```python
from build123d import *

# Parameters (mm, degrees)
SKETCH_1_W = 52
SKETCH_1_H = 6.25
SKETCH_4_W = 52
SKETCH_4_H = 4.25


with BuildPart() as part:
    # ｽｹｯﾁ1 → 回転1 (revolve)
    with BuildSketch(Plane.XY, mode=Mode.PRIVATE) as revolve_1_sk:
        with Locations((26, 3.125)):
            Rectangle(SKETCH_1_W, SKETCH_1_H)
    revolve(revolve_1_sk.sketch.rotate(Axis((500, 0, 0), (-1, 0, 0)), 270), axis=Axis((500, 0, 0), (-1, 0, 0)))

    # ｽｹｯﾁ2 → ｶｯﾄ - 回転1 (revolve, cut)
    with BuildSketch(Plane.XY, mode=Mode.PRIVATE) as cut_revolve_1_sk:
        Polygon((51.8, 6.25), (52, 6.05), (52, 6.25), align=None)
    revolve(cut_revolve_1_sk.sketch.rotate(Axis((104, 0, 0), (-1, 0, 0)), 270), axis=Axis((104, 0, 0), (-1, 0, 0)), mode=Mode.SUBTRACT)

    # ｽｹｯﾁ3 → ｶｯﾄ - 回転2 (revolve, cut)
    with BuildSketch(Plane.XY, mode=Mode.PRIVATE) as cut_revolve_2_sk:
        Polygon((0, 6.25), (0, 6.05), (0.2, 6.25), align=None)
    revolve(cut_revolve_2_sk.sketch.rotate(Axis((104, 0, 0), (-1, 0, 0)), 270), axis=Axis((104, 0, 0), (-1, 0, 0)), mode=Mode.SUBTRACT)

    # ｽｹｯﾁ4 → ｶｯﾄ - 回転3 (revolve, cut)
    with BuildSketch(Plane.XY, mode=Mode.PRIVATE) as cut_revolve_3_sk:
        with Locations((26, 2.125)):
            Rectangle(SKETCH_4_W, SKETCH_4_H)
    revolve(cut_revolve_3_sk.sketch.rotate(Axis((25, 0, 0), (-1, 0, 0)), 270), axis=Axis((25, 0, 0), (-1, 0, 0)), mode=Mode.SUBTRACT)

    # ｽｹｯﾁ5 → ｶｯﾄ - 回転4 (revolve, cut)
    with BuildSketch(Plane.XY, mode=Mode.PRIVATE) as cut_revolve_4_sk:
        Polygon((0, 4.45), (0, 4.25), (0.2, 4.25), align=None)
    revolve(cut_revolve_4_sk.sketch.rotate(Axis((25, 0, 0), (-1, 0, 0)), 270), axis=Axis((25, 0, 0), (-1, 0, 0)), mode=Mode.SUBTRACT)

    # ｽｹｯﾁ6 → ｶｯﾄ - 回転5 (revolve, cut)
    with BuildSketch(Plane.XY, mode=Mode.PRIVATE) as cut_revolve_5_sk:
        Polygon((51.8, 4.25), (52, 4.25), (52, 4.45), align=None)
    revolve(cut_revolve_5_sk.sketch.rotate(Axis((25, 0, 0), (-1, 0, 0)), 270), axis=Axis((25, 0, 0), (-1, 0, 0)), mode=Mode.SUBTRACT)


solid = part.part
```
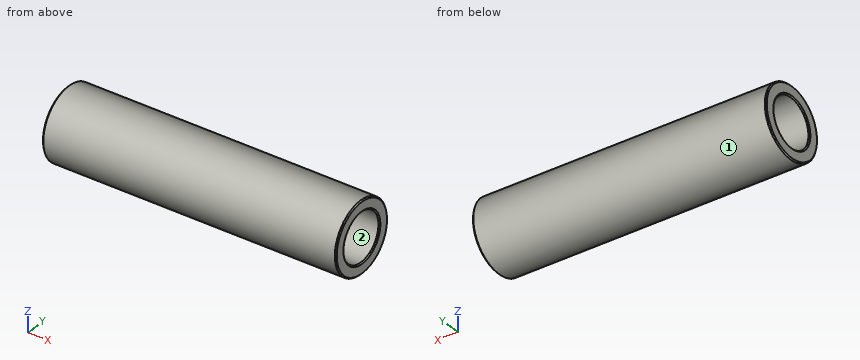
Work out the finished part from the listing and answer in its coordinate system (mm). Face numbers are marked on the shaded views. Coordinates: 2 decimals unless noted, no trailing zeros. Loops run counter-clockwise (first coordinate to the right, second up) from the corner with the lowest first, then second, coordinate; pieces in that order, holes last. Notation, with made-up numbers: (8, 30.5) -> (28, 30.5) arc R18 ccw to (28, 57.5) -> close; hole circle Ø4 at (-4.75, -31.75). An arc over 180 degrees is marked (long way). Answer as CSV lines item,"result".
Q1. Find the intervals of material crossed by probe 1 along Y at (x, z) = (22.5, 0); probe 2 along Z at (x, y) = (32.5, -0.5); probe 3 along Z at (x, y) = (47, 1.75), in increasing order.
Findings:
probe 1,"y = -6.25 to -4.25, 4.25 to 6.25"
probe 2,"z = -6.23 to -4.22, 4.22 to 6.23"
probe 3,"z = -6 to -3.87, 3.87 to 6"
Q2. For a pull along Z with two mould halves and no side action, classify the marked faces 1 and 2 as +Z half, -Z half, draft (parallel to the pull), parting line (faces both ways), or undercut.
Findings:
face 1,"parting line"
face 2,"undercut"
Q3. The part is cut by section A-A on z = 0. Write down the section's boundary in (x, y), and give its area (3 significant figures).
Findings:
outline,"(0, -6.05) -> (0.2, -6.25) -> (51.8, -6.25) -> (52, -6.05) -> (52, -4.45) -> (51.8, -4.25) -> (0.2, -4.25) -> (0, -4.45) -> close; (0, 4.45) -> (0.2, 4.25) -> (51.8, 4.25) -> (52, 4.45) -> (52, 6.05) -> (51.8, 6.25) -> (0.2, 6.25) -> (0, 6.05) -> close"
area,"208 mm²"
Q4. Each of these flat-tipped pins is pushed along its axis until it touches: pin 1 (5 mm diameter, centred on x = 6.5, z = -5, fed in from +Y); pin 2 (6 mm diameter, centred on x = 23.5, z = 3.5, fed in from +Y). Where does it stop, or does it pass through?
Findings:
pin 1,"stops at y = 5.73"
pin 2,"stops at y = 6.23"
Q5. The part is cut by section C-C on x = 36. Write down the section's boundary in (y, z), and give its area (3 significant figures).
Findings:
outline,"circle Ø12.5 at (0, 0); hole circle Ø8.5 at (0, 0)"
area,"66.0 mm²"
